from build123d import *

# Parameters (mm, degrees)
SKETCH1_W           = 101.6
SKETCH1_H           = 139.7
BOSS_EXTRUDE1_DEPTH = 6.35
CUT_EXTRUDE1_DEPTH  = 92.800885072
SKETCH4_W           = 76.2
SKETCH4_H           = 7.62
CUT_EXTRUDE2_DEPTH  = 92.800885072
SKETCH7_R           = 1.905
CUT_EXTRUDE3_DEPTH  = 92.800885072


with BuildPart() as part:
    # Sketch1 → Boss-Extrude1 (new body)
    with BuildSketch(Plane(origin=(0, 0, 0), x_dir=(1, 0, 0), z_dir=(0, 1, 0))):
        with Locations((0, 6.35)):
            Rectangle(SKETCH1_W, SKETCH1_H)
    extrude(amount=BOSS_EXTRUDE1_DEPTH)

    # Sketch3 → Cut-Extrude1 (cut, through all)
    with BuildSketch(Plane(origin=(0, 6.35, 0), x_dir=(1, 0, 0), z_dir=(0, 1, 0))):
        with BuildLine():
            Line((-1.486564617, 31.962640907), (30.263435383, 59.140640907))
            ThreePointArc((30.263435383, 59.140640907), (33.486640907, 58.890564617), (33.236564617, 55.667359093))
            Line((33.236564617, 55.667359093), (1.486564617, 28.489359093))
            ThreePointArc((1.486564617, 28.489359093), (-1.736640907, 28.739435383), (-1.486564617, 31.962640907))
        make_face()
        with BuildLine():
            Line((1.486564617, -31.962640907), (-30.263435383, -59.140640907))
            ThreePointArc((-30.263435383, -59.140640907), (-33.486640907, -58.890564617), (-33.236564617, -55.667359093))
            Line((-33.236564617, -55.667359093), (-1.486564617, -28.489359093))
            ThreePointArc((-1.486564617, -28.489359093), (1.736640907, -28.739435383), (1.486564617, -31.962640907))
        make_face()
    extrude(amount=-CUT_EXTRUDE1_DEPTH, mode=Mode.SUBTRACT)

    # Sketch4 → Cut-Extrude2 (cut, through all)
    with BuildSketch(Plane(origin=(0, 6.35, 0), x_dir=(1, 0, 0), z_dir=(0, 1, 0))):
        with Locations((0, 68.58)):
            Rectangle(SKETCH4_W, SKETCH4_H)
    extrude(amount=-CUT_EXTRUDE2_DEPTH, mode=Mode.SUBTRACT)

    # Sketch7 → Cut-Extrude3 (cut, through all)
    with BuildSketch(Plane(origin=(0, 6.35, 0), x_dir=(1, 0, 0), z_dir=(0, 1, 0))):
        with Locations(Location((-43.18, 68.58, 0), (0, 0, 270))):
            Circle(SKETCH7_R)
        with Locations(Location((43.18, 68.58, 0), (0, 0, 90))):
            Circle(SKETCH7_R)
        with Locations(Location((-43.18, -55.88, 0), (0, 0, 270))):
            Circle(SKETCH7_R)
        with Locations(Location((17.78, -55.88, 0), (0, 0, 270))):
            Circle(SKETCH7_R)
        with Locations(Location((43.18, -30.48, 0), (0, 0, 90))):
            Circle(SKETCH7_R)
    extrude(amount=-CUT_EXTRUDE3_DEPTH, mode=Mode.SUBTRACT)


solid = part.part
The model under review builds one solid part; all positions refer to its coordinate system, in mm. A direction names the side the tool comes from. Coordinates: 2 decimals unless noted, no trailing zeros. Loops run counter-clockwise (first coordinate to the right, second up) from the corner with the lowest first, then second, coordinate; pieces in that order, holes last. Notation, with made-up numbers: (50, -8.75) -> (61, -8.75) arc R13 cw to (61, 16.25) -> close; hole circle Ø5 at (30, 86). An arc over 180 degrees is marked (long way). Use a Markdown table: item, result. Add a question column.
1. Add section B-B on y = 3. Give the number of separate pieces and of enclosed holes in the cut face, plus the area to 3 significant figures.
2. Machinability: for faces 5 (the face through (-1, 0, -7)), 6 (the face through (-1, 3, -64.77)), which of the approach directions +Z, -Z, +X, -X, +Y, -Y give a long, thin tool a straight path to every point of the face, cutting with its end or side? Answer none if there is none.
3. Add section D-D on x = -31.75. Write out the cut boundary in (y, z), plus the area to 3 significant figures.
4. Draft analysis for pull direction X (two halves, no side actions). For faces 1 (the face through (-17.584, 3.219, 42.269)), 2 (the face through (-1, 3, -76.2)), 3 (the face through (-42.608, 3.219, -66.763)), 4 (the face through (50.8, 3, -5)), state which applies: pulls with the +X half, pulls with the -X half, needs draft (parallel to the pull), parting line crosses it, or undercut.
5. To check wall thickness, follow line 1 (Z direction, x = 43.18, y = 4) (3 decimals); line 2 (X direction, y = 2.25, z = -68.58) (3 decimals); line 3 (X direction, y = 3.5, z = 30.48) (3 decimals). State the ranges of each line that lie inside material, in increasing order.
6. Add section C-C on z = -68.58. Write out the cut boundary in (x, y) (3 decimals), plus the area to 3 significant figures.
7. Add section A-A on x = 36.5. Write out the cut boundary in (y, z), plus the area to 3 significant figures.
Returned:
| question | item | result |
|---|---|---|
| 1 | separate pieces | 1 |
| 1 | enclosed holes | 8 |
| 1 | area | 13,100 mm² |
| 2 | face 5 | +Z, -Z, +X, -X, -Y |
| 2 | face 6 | +Y, -Y |
| 3 | outline | (0, -76.2) -> (6.35, -76.2) -> (6.35, -72.39) -> (0, -72.39) -> close; (0, -64.77) -> (6.35, -64.77) -> (6.35, 54.39) -> (0, 54.39) -> close; (0, 59.69) -> (6.35, 59.69) -> (6.35, 63.5) -> (0, 63.5) -> close |
| 3 | area | 805 mm² |
| 4 | face 1 | undercut |
| 4 | face 2 | needs draft |
| 4 | face 3 | undercut |
| 4 | face 4 | pulls with the +X half |
| 5 | line 1 | z = -76.2 to -70.485, -66.675 to 28.575, 32.385 to 63.5 |
| 5 | line 2 | x = -50.8 to -45.085, -41.275 to -38.1, 38.1 to 41.275, 45.085 to 50.8 |
| 5 | line 3 | x = -50.8 to -3.812, 2.272 to 41.275, 45.085 to 50.8 |
| 6 | outline | (-50.8, 0) -> (-45.085, 0) -> (-45.085, 6.35) -> (-50.8, 6.35) -> close; (-41.275, 0) -> (-38.1, 0) -> (-38.1, 6.35) -> (-41.275, 6.35) -> close; (38.1, 0) -> (41.275, 0) -> (41.275, 6.35) -> (38.1, 6.35) -> close; (45.085, 0) -> (50.8, 0) -> (50.8, 6.35) -> (45.085, 6.35) -> close |
| 6 | area | 113 mm² |
| 7 | outline | (0, -76.2) -> (6.35, -76.2) -> (6.35, -72.39) -> (0, -72.39) -> close; (0, -64.77) -> (6.35, -64.77) -> (6.35, 63.5) -> (0, 63.5) -> close |
| 7 | area | 839 mm² |
